Source: three-view drawing plus pictorial views. Frame: mm from the lowest corner of the part. A direction names the side the tool comes from. Round coordinates to 2 decimals unless told otherwise and drop trailing zeros. Write each loop counter-clockwise with the first axis right and the second up, starting at its lowest first coordinate (ties: lowest second). Pieces come first, ordered by that corner, then holes. Notation, with made-up numbers: (64.5, 3.25) -> (68.5, 3.25) arc R23 ccw to (68.5, 16.25) -> close; hole circle Ø6 at (-18, 53). An arc over 180 degrees is marked (long way). Put each result on its own line as item: value.
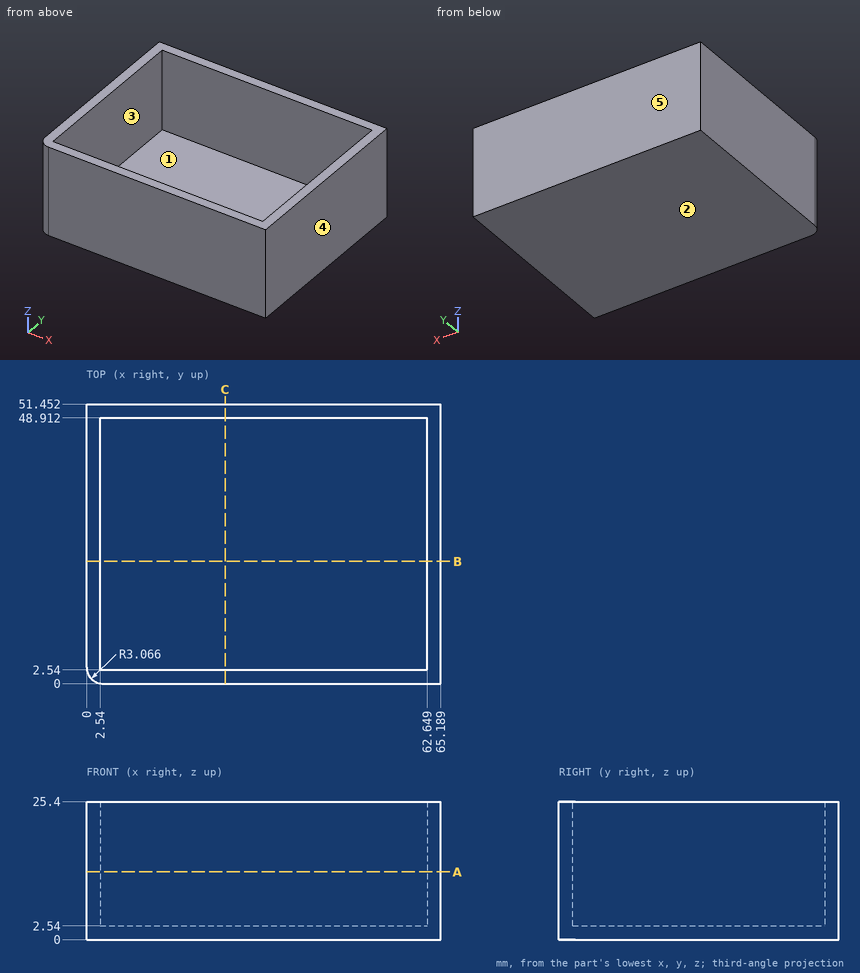
Q1. Cut plane C-C on x = 25.5. Output: boundary loops of the cut face in (y, z), and give its area (3 significant figures).
Ans:
outline: (0, 0) -> (51.45, 0) -> (51.45, 25.4) -> (48.91, 25.4) -> (48.91, 2.54) -> (2.54, 2.54) -> (2.54, 25.4) -> (0, 25.4) -> close
area: 247 mm^2
Q2. Cut plane B-B on y = 22.5. Output: boundary loops of the cut face in (x, z), and give its area (3 significant figures).
Ans:
outline: (0, 0) -> (65.19, 0) -> (65.19, 25.4) -> (62.65, 25.4) -> (62.65, 2.54) -> (2.54, 2.54) -> (2.54, 25.4) -> (0, 25.4) -> close
area: 282 mm^2
Q3. Reachability of the marked faces 1 and 2 from +Z, -Z, +X, -X, +Y, -Y: full face, straight path, thin tool, end or side. Return the list, or none.
Ans:
face 1: +Z
face 2: -Z, +X, -X, +Y, -Y
Q4. Draft query along X for the marked faces 3, 4 and 5. Return one class per face: +X half, -X half, draft (parallel to the pull), parting line (faces both ways), or undercut.
Ans:
face 3: undercut
face 4: +X half
face 5: draft
Q5. Cut plane A-A on z = 12.5. Output: boundary loops of the cut face in (x, y).
Ans:
outline: (0, 3.07) arc R3.07 ccw to (3.07, 0) -> (65.19, 0) -> (65.19, 51.45) -> (0, 51.45) -> close; hole (2.54, 2.54) -> (62.65, 2.54) -> (62.65, 48.91) -> (2.54, 48.91) -> close
Q6. Material intervals for line 1 (X direction, y = 6, z = 13.5); line 2 (Y direction, x = 39.5, z = 13); line 3 (Z direction, x = 18.5, y = 41), sorted ascending. Write a range as [from, to].
Ans:
line 1: x = [0, 2.54], [62.65, 65.19]
line 2: y = [0, 2.54], [48.91, 51.45]
line 3: z = [0, 2.54]
Q7. Pin query (flat end, axial travel): pin 1 (10 mm diameter, centred on x = 15, y = 19, fed in from -Z); pin 2 (3 mm diameter, centred on x = 44, y = 33.5, fed in from +Z). Return the tip coordinate at first contact, or that it passes through.
Ans:
pin 1: stops at z = 0
pin 2: stops at z = 2.54
